For this review, take the finished solid that the model builds, in its own axes (mm). Round coordinates to 2 decimals unless told otherwise and drop trailing zeros. Loops run counter-clockwise (first coordinate to the right, second up) from the corner with the lowest first, then second, coordinate; pieces in that order, holes last. Notation, with made-up numbers: M 51.25,51 L 94.25,51 A23 ccw 94.25,69 Z; hole C 68,-8.5 d7. An arc over 180 degrees is marked long. One line per question, with ' | ' between items. Start each with the question number.
1) For pin 1 Ø12 at (x, y) = (-59, -51.5) entering from -Z; pin 2 Ø8 at (x, y) = (-48.5, -59) entering from -Z; pin 3 Ø1 at (x, z) = (1, 1) entering from -Y; pin 4 Ø6 at (x, y) = (-28.5, -26) entering from -Z, all flat-tipped, find the tip position at first contact; note any pin that passes through.
2) We need section A-A (z = 30). Give the boundary of the cut face in (x, y), and give its area (3 significant figures).
3) We need section B-B (y = -11). Give the boundary of the cut face in (x, z).
Autodesk Inventor part; units mm, degrees
ref_plane "Arbeitsebene1" through (0, 0, 3) normal (-0.7071068, 0.7071068, 0) x (0.7071068, 0.7071068, 0)
ref_plane "Arbeitsebene2" through (0, 0, 3) normal (0, 0.8564105, 0.5162955) x (-0.4587597, -0.4587597, 0.7609724)
ref_plane "YZ Plane" through (0, 0, 0) normal (1, 0, 0) x (0, 1, 0)
sketch "Skizze1" plane through (0, 0, 0) normal (0, 0, 1) x (1, 0, 0)
  line L0 (0, 0) -> (2, 0)
  line L1 (2, 0) -> (2, 2)
  line L2 (2, 2) -> (0, 2)
  line L3 (0, 2) -> (0, 0)
  dimension "d0" = 2
  dimension "d1" = 2
extrude "Extrusion1" add sketch "Skizze1" along normal blind 3
sketch "Skizze2" plane through (0, 0, 3) normal (0, 0, 1) x (1, 0, 0)
  point P0 (0, 0)
ref_plane "Arbeitsebene1" through (0, 0, 3) normal (-0.7071068, 0.7071068, 0) x (0.7071068, 0.7071068, 0)
sketch "Skizze3" plane through (0, 0, 3) normal (-0.7071068, 0.7071068, 0) x (0.7071068, 0.7071068, 0)
  line L0 (0, 0) -> (1.4142, 0)
  line L1 (0, 0) -> (-112.5245, -131.9823)
  line L2 (0, 0) -> (173.439, 0) construction
  line L3 (2.8284, 3) -> (2.8284, 0)
  line L4 (2.8284, 0) -> (-109.6961, -131.9823)
  line L5 (2.8284, 0) -> (176.2674, 0) construction
  line L6 (-109.6961, -131.9823) -> (-112.5245, -131.9823)
  line L7 (1.4142, 0) -> (2.8284, 0)
  line L8 (2.8284, 0) -> (0, 0)
  point P0 (0, 3)
  dimension "d4" = 173.439
  dimension "d5" = 130.45
  dimension "d6" = 173.439
  dimension "d7" = 130.45
ref_plane "Arbeitsebene2" through (0, 0, 3) normal (0, 0.8564105, 0.5162955) x (-0.4587597, -0.4587597, 0.7609724)
sketch "Skizze4" plane through (0, 0, 3) normal (0, 0.8564105, 0.5162955) x (-0.4587597, -0.4587597, 0.7609724)
  line L0 (0, 0) -> (-0.9175, 1.7771)
  line L1 (0, 0) -> (-0.9175, 1.7771)
  line L2 (-0.9175, 1.7771) -> (172.5215, 1.7771)
  line L3 (172.5215, 1.7771) -> (173.439, 0)
  line L4 (173.439, 0) -> (0, 0)
  point P0 (-2.2829, -1.1787)
  dimension "d9" = 173.439
extrude "Extrusion2" add sketch "Skizze4" along normal blind 2
sketch "Skizze5" plane through (-77.5668, -79.5668, 134.9823) normal (0.8885604, -0.2368556, 0.3928866) x (0.4587597, 0.4587597, -0.7609724)
  line L0 (172.5215, 0) -> (-0.9175, 0)
  line L1 (0.0005, 0) -> (1.3553, 2)
  line L2 (0, 2) -> (173.439, 2)
  line L3 (1.3553, 2) -> (0, 2)
  line L4 (0, 0) -> (0, 2)
  line L5 (0, 2) -> (0, 0)
  point P0 (174.8044, -1.5489)
sketch "Skizze6" plane through (0, 0, 3) normal (0, -0.8564105, -0.5162955) x (0.8885604, -0.2368556, 0.3928866)
  line L0 (0, 0) -> (0, 173.439)
  line L1 (1.7771, 172.5215) -> (0, 173.439)
  point P0 (-1.1787, -2.2829)
sketch "Skizze7" plane through (0, 1.7128, 4.0326) normal (0, 0.8564105, 0.5162955) x (0.8885604, -0.2368556, 0.3928866)
  line L0 (0, 0) -> (0, -173.439)
  line L1 (0, -172.1027) -> (1.781, -171.1647)
  point P0 (-1.1787, 2.2829)
sketch "Skizze8" plane through (0, 0, 3) normal (-0.8885604, 0.2368556, -0.3928866) x (-0.4587597, -0.4587597, 0.7609724)
  line L0 (0, 2) -> (173.439, 2)
  line L1 (0, 0) -> (173.439, 0)
  line L2 (172.1026, 2) -> (173.439, 0)
  point P0 (-2.2829, -1.5489)
chamfer "Fase1" distance 1.1929 distance2 2 1 edges at (-78.5668, -77.854, 136.0149) measured on face at (-25.1889, -24.8095, 48.0267)
ref_plane "Arbeitsebene3" through (2, 0, 3) normal (-1, 0, 0) x (0, 0.8564105, 0.5162955)
sketch "Skizze12" plane through (2, 0, 3) normal (-1, 0, 0) x (0, 0.8564105, 0.5162955)
  line L0 (0, 0) -> (1.7128, 1.0326)
  line L1 (0, 0) -> (2, 0)
  line L2 (-1.5489, 2.5692) -> (0, 0)
  line L3 (0, 0) -> (1.7128, 1.0326)
  line L4 (2, 0) -> (1.7128, 1.0326)
extrude "Extrusion6" add sketch "Skizze12" along normal blind 2
properties part number "FOVStick"
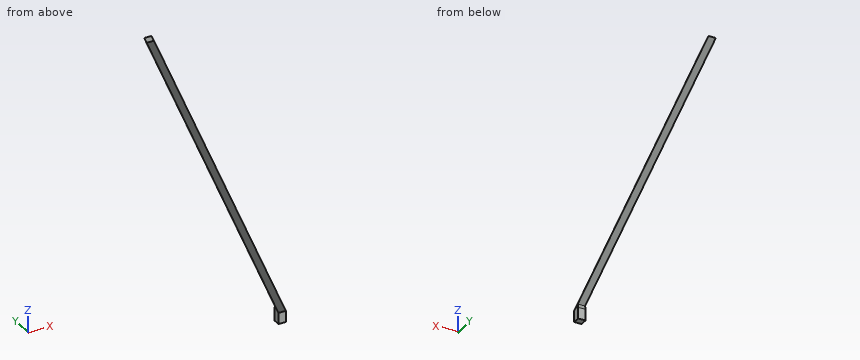
Answers below:
1) pin 1: z = 91.34 | pin 2: through | pin 3: y = 0 | pin 4: z = 45.36
2) outline: M -16.28,-16.28 L -14.28,-16.28 L -13.65,-13.94 L -15.65,-13.94 Z | area: 4.67 mm^2
3) outline: M -12.71,25.12 L -11,21.25 L -9,21.25 L -10.71,25.12 Z
